```python
from build123d import *

# Parameters (mm, degrees)
F1_DEPTH = 140


with BuildPart() as f1:
    # F0 (on Front) → F1 (new body)
    with BuildSketch(Plane.XZ):
        with BuildLine():
            Line((-5, 0), (0, 0))
            Line((0, 0), (5, 0))
            Line((5, 0), (15.905888, 18.889553))
            ThreePointArc((15.905888, 18.889553), (14.648043, 23.212289), (10.347496, 21.880553))
            Line((10.347496, 21.880553), (10.240284, 21.650635))
            Line((10.240284, 21.650635), (1.99989, 3.979054))
            Line((1.99989, 3.979054), (0, 4))
            Line((0, 4), (-1.99989, 3.979054))
            Line((-1.99989, 3.979054), (-10.240284, 21.650635))
            Line((-10.240284, 21.650635), (-10.347496, 21.880553))
            ThreePointArc((-10.347496, 21.880553), (-14.648043, 23.212289), (-15.905888, 18.889553))
            Line((-15.905888, 18.889553), (-5, 0))
        make_face()
        with BuildLine():
            Line((10.240284, 21.650635), (10.347496, 21.880553))
            ThreePointArc((10.347496, 21.880553), (10.29158, 21.766671), (10.240284, 21.650635))
        make_face()
        with BuildLine():
            ThreePointArc((-10.240284, 21.650635), (-10.29158, 21.766671), (-10.347496, 21.880553))
            Line((-10.347496, 21.880553), (-10.240284, 21.650635))
        make_face()
    extrude(amount=F1_DEPTH)


solid = f1.part
```
Verification items for the finished model (mm, model axes). A direction names the side the tool comes from. Give positions to 0.01 mm unless a question says otherwise; leave off trailing zeros. Order: outer loops, then holes, each group sorted by start corner. A loop starts at its lowest first (then second) coordinate and runs counter-clockwise, first axis right, second up. Notation, with made-up numbers: M -38.5,48 L 13.5,48 A30 ccw 13.5,85 Z; hole C 66.5,55.25 d1. An arc over 180 degrees is marked long. Return JSON: item names as keys, results as strings. Group by question number.
1) Section check D-D on z = 2. Record the cut outline in (x, y), and give its area (3 significant figures).
2) Section check B-B on y = -113. Record the cut outline in (x, z).
3) Section check C-C on x = 14. Record the cut outline in (y, z).
4) Access from +Z, -Z, +X, -X, +Y, -Y to the whole of each face (thin tool, end or side, straight path). Record for faces 4 (the face through (14.71, -69.02, 23.18)), 5 (the face through (6.18, -69.02, 12.94)).
5) Mould release check, pull along X, two halves, no side actions. Record for faces 1 (the face through (-4, -140, 7)), 2 (the face through (10.377, -69.02, 9.313)), 3 (the face through (-6.06, -69.02, 12.69)): pulls with the +X half, pulls with the -X half, needs draft (parallel to the pull), parting line crosses it, or undercut.
6) Go/stop test with flat-tipped pins: pin 1 Ø5 at (x, z) = (5, 17.5) entering from -Y; pin 2 Ø5 at (y, z) = (-42, 10.5) entering from +X; pin 3 Ø8 at (y, z) = (-20, 13) entering from -X; pin 4 Ø8 at (x, y) = (6.5, -98) entering from +Z. Record where each tip stops, or that it passes through.
7) Section check A-A on z = 8. Record the cut outline in (x, y), and give its area (3 significant figures).
8) Scan lines: line 1 (X direction, y = -69, z = 19.75); line 2 (Z direction, x = -2, y = -23.5); line 3 (X direction, y = -13, z = 18.75). Record each from-to range of solid material in increasing order.
Answer block:
{
 "1": {"outline": "M -6.15,-140 L 6.15,-140 L 6.15,0 L -6.15,0 Z", "area": "1,720 mm^2"},
 "2": {"outline": "M -15.91,18.89 L -5,0 L 5,0 L 15.91,18.89 A3.16 ccw long 10.35,21.88 A3.16 ccw 10.24,21.65 L 2,3.98 L 0,4 L -2,3.98 L -10.24,21.65 A3.16 ccw -10.35,21.88 A3.16 ccw long Z"},
 "3": {"outline": "M -140,15.59 L 0,15.59 L 0,23.47 L -140,23.47 Z"},
 "4": {"face 4": "+Y, -Y", "face 5": "+Z, +Y, -Y"},
 "5": {"face 1": "needs draft", "face 2": "pulls with the +X half", "face 3": "undercut"},
 "6": {"pin 1": "passes through", "pin 2": "stops at x = 12.51", "pin 3": "stops at x = -14.81", "pin 4": "stops at z = 22.14"},
 "7": {"outline": "M -9.62,-140 L -3.87,-140 L -3.87,0 L -9.62,0 Z; M 3.87,-140 L 9.62,-140 L 9.62,0 L 3.87,0 Z", "area": "1,610 mm^2"},
 "8": {"line 1": "x = -16.23 to -9.35, 9.35 to 16.23", "line 2": "z = 0 to 3.98", "line 3": "x = -15.83 to -8.89, 8.89 to 15.83"}
}
